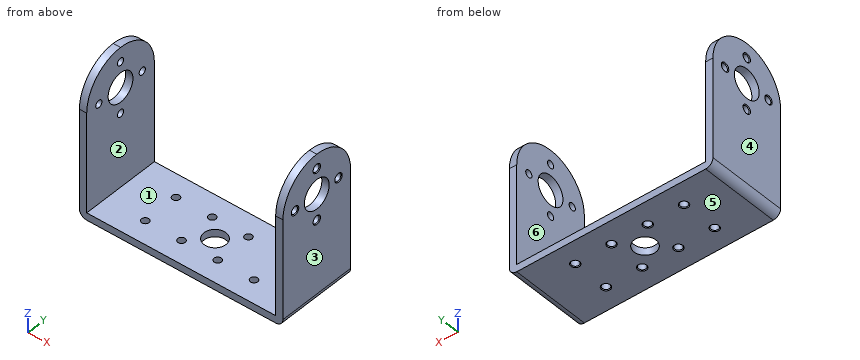
Autodesk Inventor part; units mm, degrees
ref_plane "YZ Plane" through (0, 0, 0) normal (1, 0, 0) x (0, 1, 0)
ref_plane "XZ Plane" through (0, 0, 0) normal (0, 1, 0) x (-1, 0, 0)
ref_plane "XY Plane" through (0, 0, 0) normal (0, 0, 1) x (1, 0, 0)
sketch "Sketch1" plane through (0, 0, 0) normal (0, 0, 1) x (1, 0, 0)
  line L0 (0, 0) -> (55.6, 0)
  line L1 (55.6, 0) -> (55.6, 21.8)
  line L2 (55.6, 21.8) -> (0, 21.8)
  line L3 (0, 21.8) -> (0, 0)
  dimension "d2" = 21.8
extrude "Extrusion1" add sketch "Sketch1" along normal blind 2
sketch "Sketch2" plane through (0, 0, 2) normal (0, 0, 1) x (1, 0, 0)
  line L0 (0, 21.8) -> (0, 0)
  line L1 (55.6, 21.8) -> (0, 21.8)
  line L2 (0, 0) -> (2, 0)
  line L3 (2, 0) -> (2, 21.8)
  line L4 (2, 21.8) -> (0, 21.8)
  line L5 (0, 21.8) -> (0, 0)
  line L6 (0, 0) -> (55.6, 0)
  line L7 (55.6, 21.8) -> (53.6, 21.8)
  line L8 (53.6, 21.8) -> (53.6, 0)
  line L9 (53.6, 0) -> (55.6, 0)
  line L10 (55.6, 0) -> (55.6, 21.8)
  dimension "d5" = 2
  dimension "d6" = 2
extrude "Extrusion2" add sketch "Sketch2" along normal blind 38 contours L1 L3 L2 L0 | L1 L10 L6 L8
fillet "Fillet1" radius 10.9 4 edges at (54.6, 21.8, 40) (54.6, 0, 40) (1, 0, 40) (1, 21.8, 40)
fillet "Fillet2" radius 2 2 edges at (55.6, 10.9, 0) (0, 10.9, 0)
sketch "Sketch3" plane through (55.6, 10.9, 29.1) normal (1, 0, 0) x (0, 0, -1)
  arc A0 (0, 10.9) -> (0, -10.9) centre (0, 0) ccw
  circle A1 centre (0, 0) radius 1
  point P0 (29.1, -10.9)
  dimension "d12" = 2
hole "Hole1" at (55.6, 10.9, 29.1) direction (-1, 0, 0) diameter 8 depth 70
sketch "Sketch4" plane through (55.6, 10.9, 29.1) normal (1, 0, 0) x (0, 0, -1)
  circle A0 centre (0, 0) radius 4
  circle A1 centre (0, 0) radius 7
  circle A2 centre (0, 7) radius 1
  circle A3 centre (-7, 0) radius 1
  circle A4 centre (0, -7) radius 1
  circle A5 centre (7, 0) radius 1
  point P0 (29.1, -10.9)
  dimension "d22" = 14
  dimension "d23" = 2
  dimension "d26" = 360
hole "Hole2" at (55.6, 17.9, 29.1) at (55.6, 10.9, 22.1) at (55.6, 3.9, 29.1) at (55.6, 10.9, 36.1) direction (-1, 0, 0) diameter 2 depth 70
thread "Thread2"
thread "Thread3"
thread "Thread4"
thread "Thread5"
thread "Thread7"
thread "Thread8"
thread "Thread9"
thread "Thread10"
chamfer "Chamfer2" distance 0.2 angle 45 8 edges at (55.6, 10.9, 37.1) (55.6, 3.9, 30.1) (55.6, 10.9, 23.1) (55.6, 17.9, 30.1) (0, 10.9, 37.1) (0, 17.9, 30.1) (0, 3.9, 30.1) (0, 10.9, 23.1)
sketch "Sketch5" plane through (0, 0, 0) normal (0, 0, -1) x (-1, 0, 0)
  line L0 (-53.6, 21.8) -> (-2, 21.8)
  line L1 (-27.8, 21.8) -> (-27.8, 0)
  circle A0 centre (-27.8, 10.9) radius 3
  circle A1 centre (-27.8, 10.9) radius 7
  line L2 (-27.8, 10.9) -> (-40.3616, 10.9)
  line L3 (-27.8, 10.9) -> (-34.2529, 17.3529)
  line L4 (-27.8, 10.9) -> (-18.6742, 10.9) construction
  circle A2 centre (-32.7497, 15.8497) radius 1
  circle A3 centre (-32.7497, 5.9503) radius 1
  circle A4 centre (-22.8503, 5.9503) radius 1
  circle A5 centre (-22.8503, 15.8497) radius 1
  line L5 (-32.7497, 15.8497) -> (-42.6487, 15.8497)
  circle A6 centre (-42.6487, 15.8497) radius 1
  circle A7 centre (-42.6487, 5.9503) radius 1
  line L6 (-22.8503, 15.8497) -> (-12.9513, 15.8497)
  circle A8 centre (-12.9513, 15.8497) radius 1
  circle A9 centre (-12.9513, 5.9503) radius 1
  point P0 (0, 0)
  dimension "d60" = 14
  dimension "d59" = 6
  dimension "d61" = 135
  dimension "d62" = 2
  dimension "d65" = 360
  dimension "d67" = 9.899
  dimension "d68" = 2
  dimension "d69" = 2
  dimension "d70" = 9.899
  dimension "d71" = 2
  dimension "d72" = 2
hole "Hole3" at (42.6487, 15.8497, 0) at (32.7497, 15.8497, 0) at (22.8503, 15.8497, 0) at (12.9513, 15.8497, 0) at (12.9513, 5.9503, 0) at (22.8503, 5.9503, 0) at (32.7497, 5.9503, 0) at (42.6487, 5.9503, 0) direction (0, 0, 1) diameter 2 depth 3
sketch "Sketch6" plane through (0, 0, 0) normal (0, 0, -1) x (-1, 0, 0)
  line L0 (-2, 0) -> (-53.6, 0)
  line L1 (-27.8, 0) -> (-27.8, 21.8)
  line L2 (-53.6, 21.8) -> (-2, 21.8)
  circle A0 centre (-27.8, 10.9) radius 3
  point P0 (0, 0)
  dimension "d80" = 6
hole "Hole4" at (27.8, 10.9, 0) direction (0, 0, 1) diameter 6 depth 3
chamfer "Chamfer3" distance 0.2 angle 45 8 edges at (12.9513, 4.9503, 0) (22.8503, 4.9503, 0) (32.7497, 4.9503, 0) (42.6487, 4.9503, 0) (12.9513, 14.8497, 0) (22.8503, 14.8497, 0) (32.7497, 14.8497, 0) (42.6487, 14.8497, 0)
CAD build for the part. Positions are in the model's coordinates, mm. Face numbers are marked on the shaded views. A direction names the side the tool comes from. Round coordinates to 2 decimals unless told otherwise and drop trailing zeros. Write each loop counter-clockwise with the first axis right and the second up, starting at its lowest first coordinate (ties: lowest second). Pieces come first, ordered by that corner, then holes. Notation, with made-up numbers: M 20.5,82.5 L 43.5,82.5 A15 cw 43.5,97.5 Z; hole C 37,57 d8. An arc over 180 degrees is marked long. Use a Markdown table: item, result. Add a question column.
1. 3-axis set-ups, long thin cutter, end or side, ignore diameter. For the marked faces 5 and 6: which of +Z, -Z, +X, -X, +Y, -Y reach the whole face in a straight line?
2. Drill centre lines: probe 1 along Y at (x, z) = (1, 22); probe 2 along X at (y, z) = (2.25, 29); probe 3 along Z at (x, y) = (54.8, 10.9). Where is each one in solid material? Low to high.
3. Flat gauge pin, fed straight in: P1, Ø4, axis at x = 11, y = 17.5, coming from the +Z side. Where does the tip first touch, or does it go through?
4. Slice it at A-A on z = 4.5. Give the cut face in (x, y).
5. Pull direction X, two halves, no side cores. Call the marked faces 1, 2, 3 and 4: released by +X, released by -X, zero draft, split by the parting line, or undercut.
6. Slice it at D-D on y = 17.9. Give the cut face in (x, z), then the cut area to 3 significant figures.
7. Slice it at B-B on x = 27.8. Give the cut face in (y, z), then the cut area to 3 significant figures.
8. Slice it at C-C on z = 22.1. Give the cut face in (x, y), then the cut area to 3 significant figures.
Reply:
| question | item | result |
|---|---|---|
| 1 | face 5 | -Z, +X, -X, +Y, -Y |
| 1 | face 6 | +Z, +Y, -Y |
| 2 | probe 1 | y = 0 to 9.91, 11.89 to 21.8 |
| 2 | probe 2 | x = 0 to 2, 53.6 to 55.6 |
| 2 | probe 3 | z = 0.4 to 21.1, 23.1 to 25.1, 33.1 to 35.1, 37.1 to 40 |
| 3 | P1 | stops at z = 2 |
| 4 | outline | M 0,0 L 2,0 L 2,21.8 L 0,21.8 Z; M 53.6,0 L 55.6,0 L 55.6,21.8 L 53.6,21.8 Z |
| 5 | face 1 | undercut |
| 5 | face 2 | undercut |
| 5 | face 3 | released by +X |
| 5 | face 4 | released by -X |
| 6 | outline | M 0,2 A2 ccw 2,0 L 53.6,0 A2 ccw 55.6,2 L 55.6,27.9 L 55.4,28.1 L 53.6,28.1 L 53.6,2 L 2,2 L 2,28.1 L 0.2,28.1 L 0,27.9 Z; M 0,30.3 L 0.2,30.1 L 2,30.1 L 2,37.46 L 0,37.46 Z; M 53.6,30.1 L 55.4,30.1 L 55.6,30.3 L 55.6,37.46 L 53.6,37.46 Z |
| 6 | area | 243 mm^2 |
| 7 | outline | M 0,0 L 7.9,0 L 7.9,2 L 0,2 Z; M 13.9,0 L 21.8,0 L 21.8,2 L 13.9,2 Z |
| 7 | area | 31.6 mm^2 |
| 8 | outline | M 0,0 L 2,0 L 2,9.9 L 0.2,9.9 L 0,9.7 Z; M 0,12.1 L 0.2,11.9 L 2,11.9 L 2,21.8 L 0,21.8 Z; M 53.6,0 L 55.6,0 L 55.6,9.7 L 55.4,9.9 L 53.6,9.9 Z; M 53.6,11.9 L 55.4,11.9 L 55.6,12.1 L 55.6,21.8 L 53.6,21.8 Z |
| 8 | area | 79.1 mm^2 |
